```python
from build123d import *

# Parameters (mm, degrees)
SKETCH2_R          = 12.5
CUT_EXTRUDE1_DEPTH = 116.779963724
CIRPATTERN1_COUNT  = 4


with BuildPart() as part:
    # Sketch1 → Revolve1 (revolve)
    with BuildSketch(Plane.XY, mode=Mode.PRIVATE) as revolve1_sk:
        Polygon((0, 0), (30, 0), (30, 50), (25, 50), (25, 45), (5, 45), (5, 50), (0, 50), align=None)
    revolve(revolve1_sk.sketch.rotate(Axis((-128.92900602, -19, 0), (1, 0, 0)), 90), axis=Axis((-128.92900602, -19, 0), (1, 0, 0)))

    # Sketch2 → Cut-Extrude1 (cut, through all)
    with BuildSketch(Plane(origin=(30, 0, 0), x_dir=(0, 0, -1), z_dir=(1, 0, 0))):
        with Locations((0, 30)):
            Circle(SKETCH2_R)
    cut_extrude1 = extrude(amount=-CUT_EXTRUDE1_DEPTH, mode=Mode.SUBTRACT)

    # CirPattern1: Cut-Extrude1 ×4 about axis
    cirpattern1_axis = Axis((0, -19, 0), (1, 0, 0))
    for i in range(1, CIRPATTERN1_COUNT):
        add(cut_extrude1.rotate(cirpattern1_axis, i * 360 / CIRPATTERN1_COUNT), mode=Mode.SUBTRACT)


solid = part.part
```
The model under review builds one solid part; all positions refer to its coordinate system, in mm. A direction names the side the tool comes from. Give positions to 0.01 mm unless a question says otherwise; leave off trailing zeros. Order: outer loops, then holes, each group sorted by start corner. A loop starts at its lowest first (then second) coordinate and runs counter-clockwise, first axis right, second up. Notation, with made-up numbers: (-30.75, -13.5) - (13.25, -13.5) arc R31 cw to (13.25, 22.5) - close; hole circle Ø8 at (49, -18). An arc over 180 degrees is marked (long way). Use CSV: the item, a comma, the result in double quotes. Start each with the question number.
Q1. We need section C-C, the plane z = -59.5. Write out the cut boundary in (x, y).
Q2. Tool access review of faces 1 (the cylindrical face through (14.86, 19.94, -50.79)), 2 (the cylindrical face through (15.21, -28.92, 41.394)): name each direction out of +Z, -Z, +X, -X, +Y, -Y from which nothing blocks a thin tool from reaching the whole face with its end or side.
Q3. The part is to be moulded in two halves that separate along Y. For faces 3 (the cylindrical face through (15.21, -80.394, -1.627)), 4 (the cylindrical face through (2.46, 48.36, -14.96)), 5 (the flat face through (0, -5, 14)), 6 (the cylindrical face through (15.21, -35.021, 10.214)), say which applies: +Y half, -Y half, draft (parallel to the pull), parting line (faces both ways), or undercut.
Q4. We need section B-B, the plane z = 0. Write out the cut boundary in (x, y), and give its area (3 significant figures).
Q5. We need section A-A, the plane y = -19. Write out the cut boundary in (x, z).
Q6. We need section D-D, the plane y = 30. Write out the cut boundary in (x, z), and give its area (3 significant figures).
Q7. To check wall thickness, follow line 1 along Y through (x, z) = (7.25, 0); line 2 along X through (y, z) = (12, -58); line 3 along Y through (x, z) = (28.75, -1). State the ranges of each line that lie inside material, in increasing order. Write a range as [from, to].
Q8. Clearance check with flat-ended pins moving along their axes: pin 1 Ø1.5 at (x, y) = (3.5, -22) entering from +Z; pin 2 Ø10 at (x, y) = (22, -61.5) entering from +Z; pin 3 Ø10 at (x, z) = (4.5, -8) entering from -Y; pin 4 Ø4 at (y, z) = (-16, 24.5) entering from -X. State where each tip first meets the part, or that it passes through.
Outcome:
1,outline,"(0, -53.94) - (5, -53.94) - (5, -42.57) - (25, -42.57) - (25, -53.94) - (30, -53.94) - (30, -25.78) - (0, -25.78) - close; (0, -12.22) - (30, -12.22) - (30, 15.94) - (25, 15.94) - (25, 4.57) - (5, 4.57) - (5, 15.94) - (0, 15.94) - close"
2,face 1,"none"
2,face 2,"+X, -X"
3,face 3,"undercut"
3,face 4,"parting line"
3,face 5,"draft"
3,face 6,"undercut"
4,outline,"(0, -88) - (5, -88) - (5, -83) - (25, -83) - (25, -88) - (30, -88) - (30, -80.5) - (0, -80.5) - close; (0, -55.5) - (30, -55.5) - (30, -38) - (0, -38) - close; (0, 0) - (30, 0) - (30, 17.5) - (0, 17.5) - close; (0, 42.5) - (30, 42.5) - (30, 50) - (25, 50) - (25, 45) - (5, 45) - (5, 50) - (0, 50) - close"
4,area,"1,300 mm^2"
5,outline,"(0, -69) - (5, -69) - (5, -64) - (25, -64) - (25, -69) - (30, -69) - (30, -61.5) - (0, -61.5) - close; (0, -36.5) - (30, -36.5) - (30, -19) - (0, -19) - close; (0, 19) - (30, 19) - (30, 36.5) - (0, 36.5) - close; (0, 61.5) - (30, 61.5) - (30, 69) - (25, 69) - (25, 64) - (5, 64) - (5, 69) - (0, 69) - close"
6,outline,"(0, -48.58) - (5, -48.58) - (5, -41.17) - (25, -41.17) - (25, -48.58) - (30, -48.58) - (30, -12.5) - (0, -12.5) - close; (0, 12.5) - (30, 12.5) - (30, 48.58) - (25, 48.58) - (25, 41.17) - (5, 41.17) - (5, 48.58) - (0, 48.58) - close"
6,area,"1,870 mm^2"
7,line 1,"y = [-83, -80.5], [-55.5, -38], [0, 17.5], [42.5, 45]"
7,line 2,"x = [0, 5], [25, 30]"
7,line 3,"y = [-87.99, -80.46], [-55.54, -37.97], [-0.03, 17.54], [42.46, 49.99]"
8,pin 1,"stops at z = 68.96"
8,pin 2,"stops at z = 57.26"
8,pin 3,"stops at y = -87.93"
8,pin 4,"stops at x = 0"
